Could you check a few things on this model? Use its own coordinates, in mm. Round coordinates to 2 decimals unless told otherwise and drop trailing zeros. Answer in a Markdown table with one row per item. Add a question column.
```python
from build123d import *

# Parameters (mm, degrees)
SKETCH1_W           = 250
SKETCH1_H           = 30
BOSS_EXTRUDE1_DEPTH = 3.175
FILLET1_R           = 5
SKETCH2_R           = 2.5
CUT_EXTRUDE1_DEPTH  = 236.499640393
SKETCH3_R           = 1.625
CUT_EXTRUDE3_DEPTH  = 236.499640393
SKETCH4_R           = 1.75
CUT_EXTRUDE4_DEPTH  = 10
SKETCH5_R           = 2.125
CUT_EXTRUDE5_DEPTH  = 236.499640393


with BuildPart() as part:
    # Sketch1 → Boss-Extrude1 (new body)
    with BuildSketch(Plane(origin=(0, 0, 0), x_dir=(1, 0, 0), z_dir=(0, 1, 0))):
        with Locations((110, 0)):
            Rectangle(SKETCH1_W, SKETCH1_H)
    extrude(amount=BOSS_EXTRUDE1_DEPTH)

    # Fillet1
    fillet1_edges = [part.edges().sort_by_distance(p)[0] for p in [
        (-15, 1.5875, -15),
        (235, 1.5875, -15),
        (235, 1.5875, 15),
        (-15, 1.5875, 15),
    ]]
    fillet(fillet1_edges, radius=FILLET1_R)

    # Sketch2 → Cut-Extrude1 (cut, through all)
    with BuildSketch(Plane(origin=(0, 3.175, 0), x_dir=(1, 0, 0), z_dir=(0, 1, 0))):
        with Locations(Location((0, 0, 0), (0, 0, 270))):
            Circle(SKETCH2_R)
    extrude(amount=-CUT_EXTRUDE1_DEPTH, mode=Mode.SUBTRACT)

    # Sketch3 → Cut-Extrude3 (cut, through all)
    with BuildSketch(Plane(origin=(0, 3.175, 0), x_dir=(1, 0, 0), z_dir=(0, 1, 0))):
        with Locations(Location((7.5, 0, 0), (0, 0, 270))):
            Circle(SKETCH3_R)
        with Locations(Location((0, -7.5, 0), (0, 0, 270))):
            Circle(SKETCH3_R)
        with Locations(Location((-7.5, 0, 0), (0, 0, 270))):
            Circle(SKETCH3_R)
        with Locations(Location((0, 7.5, 0), (0, 0, 270))):
            Circle(SKETCH3_R)
    extrude(amount=-CUT_EXTRUDE3_DEPTH, mode=Mode.SUBTRACT)

    # Sketch4 → Cut-Extrude4 (cut)
    with BuildSketch(Plane(origin=(0, 3.175, 0), x_dir=(1, 0, 0), z_dir=(0, 1, 0))):
        with Locations(Location((85, -10, 0), (0, 0, 270))):
            Circle(SKETCH4_R)
        with Locations(Location((135, -10, 0), (0, 0, 270))):
            Circle(SKETCH4_R)
        with Locations(Location((135, 10, 0), (0, 0, 270))):
            Circle(SKETCH4_R)
        with Locations(Location((85, 10, 0), (0, 0, 270))):
            Circle(SKETCH4_R)
        with Locations(Location((175, -10, 0), (0, 0, 270))):
            Circle(SKETCH4_R)
        with Locations(Location((175, 10, 0), (0, 0, 270))):
            Circle(SKETCH4_R)
        with Locations(Location((45, -10, 0), (0, 0, 270))):
            Circle(SKETCH4_R)
        with Locations(Location((45, 10, 0), (0, 0, 270))):
            Circle(SKETCH4_R)
    extrude(amount=-CUT_EXTRUDE4_DEPTH, mode=Mode.SUBTRACT)

    # Sketch5 → Cut-Extrude5 (cut, through all)
    with BuildSketch(Plane(origin=(0, 3.175, 0), x_dir=(1, 0, 0), z_dir=(0, 1, 0))):
        with Locations(Location((216, 8, 0), (0, 0, 270))):
            Circle(SKETCH5_R)
        with Locations(Location((228, 8, 0), (0, 0, 90))):
            Circle(SKETCH5_R)
        with Locations(Location((228, -8, 0), (0, 0, 270))):
            Circle(SKETCH5_R)
        with Locations(Location((216, -8, 0), (0, 0, 90))):
            Circle(SKETCH5_R)
    extrude(amount=-CUT_EXTRUDE5_DEPTH, mode=Mode.SUBTRACT)


solid = part.part
```
(1) If we mould it in two halves opening along X, with no side actions, what happens to faces 1 (the face through (108, 0, 0)), 2 (the face through (233, 2, 14)), 3 (the face through (229.792, 1.61, 9.142))? For each: pulls with the +X half, pulls with the -X half, needs draft (parallel to the pull), parting line crosses it, or undercut.
(2) I need wall thicknesses on L1, parallel to Z at x = 216, y = 1.7 (3 decimals); L2, parallel to Z at x = 85, y = 1.25; L3, parallel to X at y = 0.8, z = 0 (3 decimals). Which ranges of each line are inside material? Lowest first, please.
(3) Suppose I cut it at A-A, the plane y = 2.3. State how many separate pieces and enclosed holes the cut face has, then the cut area to 3 significant figures.
Response:
| question | item | result |
|---|---|---|
| 1 | face 1 | needs draft |
| 1 | face 2 | pulls with the +X half |
| 1 | face 3 | undercut |
| 2 | L1 | -15 to -10.125, -5.875 to 5.875, 10.125 to 15 |
| 2 | L2 | -15 to -11.75, -8.25 to 8.25, 11.75 to 15 |
| 2 | L3 | -15 to -9.125, -5.875 to -2.5, 2.5 to 5.875, 9.125 to 235 |
| 3 | separate pieces | 1 |
| 3 | enclosed holes | 17 |
| 3 | area | 7,290 mm² |
